from build123d import *

# Parameters (mm, degrees)
F0_W     = 140
F0_H     = 86
F1_DEPTH = 3
F2_R     = 4
F2_R_2   = 1.5
F3_DEPTH = 15
F4_W     = 40
F4_H     = 86
F4_W_2   = 10
F4_H_2   = 12
F4_W_3   = 4
F4_H_3   = 25
F5_DEPTH = 2


with BuildPart() as f1:
    # F0 (on Front) → F1 (new body)
    with BuildSketch(Plane.XZ):
        Rectangle(F0_W, F0_H)
    extrude(amount=-F1_DEPTH)

    # F2 (on face) → F3 (join)
    with BuildSketch(Plane.XZ):
        with Locations((65.75, 38.5)):
            Circle(F2_R)
        with Locations((65.75, 38.5)):
            Circle(F2_R_2, mode=Mode.SUBTRACT)
        with Locations((-65.75, 38.5)):
            Circle(F2_R)
        with Locations((-65.75, 38.5)):
            Circle(F2_R_2, mode=Mode.SUBTRACT)
        with Locations((-65.75, -38.5)):
            Circle(F2_R)
        with Locations((-65.75, -38.5)):
            Circle(F2_R_2, mode=Mode.SUBTRACT)
        with Locations((65.75, -38.5)):
            Circle(F2_R)
        with Locations((65.75, -38.5)):
            Circle(F2_R_2, mode=Mode.SUBTRACT)
    extrude(amount=F3_DEPTH)

    # F4 (on face) → F5 (join)
    with BuildSketch(Plane(origin=(-70, 0, 0), x_dir=(0, -1, 0), z_dir=(-1, 0, 0))):
        with Locations((17, 0)):
            Rectangle(F4_W, F4_H)
        with Locations((23, -4.3)):
            Rectangle(F4_W_2, F4_H_2, mode=Mode.SUBTRACT)
        with Locations((20, 20.3)):
            Rectangle(F4_W_3, F4_H_3, mode=Mode.SUBTRACT)
    extrude(amount=F5_DEPTH)


solid = f1.part
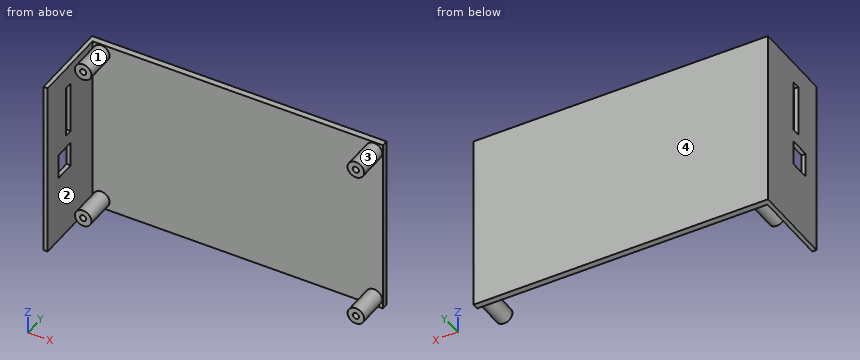
For this review, take the finished solid that the model builds, in its own axes (mm). Face numbers are marked on the shaded views. A direction names the side the tool comes from. Round coordinates to 2 decimals unless told otherwise and drop trailing zeros. Order: outer loops, then holes, each group sorted by start corner. A loop starts at its lowest first (then second) coordinate and runs counter-clockwise, first axis right, second up. Notation, with made-up numbers: M 37,57.25 L 59,57.25 A23 cw 59,96.25 Z; hole C -28.5,-5 d8. An arc over 180 degrees is marked long. Write each question's results on one line, items separated by ' | '. Start each with the question number.
1. Tool access review of the marked faces 3 and 4: name each direction out of +Z, -Z, +X, -X, +Y, -Y from which nothing blocks a thin tool from reaching the whole face with its end or side.
2. Add section C-C (x = -65.75). State the section outline as (y, z) points.
3. Add section A-A (z = 14). State the section outline as (x, y) points.
4. Clearance check with flat-ended pins moving along their axes: pin 1 Ø2.5 at (x, z) = (64, 39) entering from -Y; pin 2 Ø1 at (x, z) = (55.5, 28) entering from -Y; pin 3 Ø1 at (y, z) = (-26.5, -26) entering from +X. State where each tip first meets the part, or that it passes through.
5. To check wall thickness, follow L1, parallel to Z at x = -65.75, y = -5.75; L2, parallel to X at y = -10, z = -38; L3, parallel to Y at x = -11.5, z = -2. State the ranges of each line that lie inside material, in increasing order. Write a range as [from, to].
6. Add section B-B (z = -38.5). State the section outline as (x, y) points.
7. Add section D-D (z = -14). State the section outline as (x, y) points, then the cut area to 3 significant figures.
8. Draft analysis for pull direction Z (two halves, no side actions). For the marked faces 1 and 2, state which applies: pulls with the +Z half, pulls with the -Z half, needs draft (parallel to the pull), parting line crosses it, or undercut.
Output values:
1) face 3: -Y | face 4: +Z, -Z, +X, -X, +Y
2) outline: M -15,-42.5 L 0,-42.5 L 0,-43 L 3,-43 L 3,43 L 0,43 L 0,42.5 L -15,42.5 L -15,40 L 0,40 L 0,37 L -15,37 L -15,34.5 L 0,34.5 L 0,-34.5 L -15,-34.5 L -15,-37 L 0,-37 L 0,-40 L -15,-40 Z
3) outline: M -72,-37 L -70,-37 L -70,-22 L -72,-22 Z; M -72,-18 L -70,-18 L -70,0 L 70,0 L 70,3 L -72,3 Z
4) pin 1: y = -15 | pin 2: y = 0 | pin 3: x = -70
5) L1: [-42.5, -40], [-37, -34.5], [34.5, 37], [40, 42.5] | L2: [-72, -70], [-69.72, -67.16], [-64.34, -61.78], [61.78, 64.34], [67.16, 69.72] | L3: [0, 3]
6) outline: M -72,-37 L -70,-37 L -70,0 L -69.75,0 L -69.75,-15 L -67.25,-15 L -67.25,0 L -64.25,0 L -64.25,-15 L -61.75,-15 L -61.75,0 L 61.75,0 L 61.75,-15 L 64.25,-15 L 64.25,0 L 67.25,0 L 67.25,-15 L 69.75,-15 L 69.75,0 L 70,0 L 70,3 L -72,3 Z
7) outline: M -72,-37 L -70,-37 L -70,0 L 70,0 L 70,3 L -72,3 Z | area: 500 mm^2
8) face 1: undercut | face 2: needs draft
